Autodesk Inventor part; units mm, degrees
ref_plane "YZ Plane" through (0, 0, 0) normal (1, 0, 0) x (0, 1, 0)
ref_plane "XZ Plane" through (0, 0, 0) normal (0, 1, 0) x (-1, 0, 0)
ref_plane "XY Plane" through (0, 0, 0) normal (0, 0, 1) x (1, 0, 0)
sketch "Sketch1" plane through (0, 0, 0) normal (0, 0, 1) x (1, 0, 0)
  line L0 (0, 0) -> (25.4, 0)
  line L1 (25.4, 0) -> (25.4, 25.4)
  line L2 (25.4, 25.4) -> (0, 25.4)
  line L3 (0, 25.4) -> (0, 0)
  line L4 (3.175, 3.175) -> (22.225, 3.175)
  line L5 (22.225, 3.175) -> (22.225, 22.225)
  line L6 (22.225, 22.225) -> (3.175, 22.225)
  line L7 (3.175, 22.225) -> (3.175, 3.175)
  dimension "d0" = 25.4
  dimension "d1" = 25.4
  dimension "d2" = 19.05
  dimension "d3" = 19.05
  dimension "d4" = 3.175
  dimension "d5" = 3.175
extrude "Extrusion1" add sketch "Sketch1" along normal blind 146.05
sketch "Sketch2" plane through (0, 0, 0) normal (-1, 0, 0) x (0, 0, 1)
  line L0 (0, 25.4) -> (0, 0)
  line L1 (0, 0) -> (146.05, 0)
  point P0 (6.35, 12.7)
  point P1 (57.15, 12.7)
  dimension "d8" = 12.7
  dimension "d9" = 6.35
  dimension "d10" = 12.7
  dimension "d11" = 57.15
hole "Hole1" at (0, 12.7, 6.35) at (0, 12.7, 57.15) direction (1, 0, 0) diameter 6.35 end through all
sketch "Sketch3" plane through (25.4, 0, 0) normal (1, 0, 0) x (0, 0, -1)
  line L0 (-146.05, 0) -> (-146.05, 25.4)
  line L1 (0, 0) -> (-146.05, 0)
  point P0 (-95.25, 12.7)
  dimension "d19" = 50.8
  dimension "d20" = 12.7
hole "Hole2" at (25.4, 12.7, 95.25) direction (-1, 0, 0) diameter 17.4625 end through all
properties part number "back roller 1x1"
The model under review builds one solid part; all positions refer to its coordinate system, in mm. A direction names the side the tool comes from. Give positions to 0.01 mm unless a question says otherwise; leave off trailing zeros. Order: outer loops, then holes, each group sorted by start corner. A loop starts at its lowest first (then second) coordinate and runs counter-clockwise, first axis right, second up. Notation, with made-up numbers: M 71.5,75.5 L 111.5,75.5 A15 cw 111.5,79.5 Z; hole C 23.25,-32.5 d10. An arc over 180 degrees is marked long. Use one line per item in the form item = value. Start each with the question number.
Item 1: For faces 4 (the flat face through (13, 0, 72)), 5 (the flat face through (3.175, 13, 72)), list the 3-axis set-ups (+Z, -Z, +X, -X, +Y, -Y) from which the entire face can be reached by the end or side of a thin tool; tool diameter is ignored.
Item 2: We need section B-B on z = 95.25. Give the boundary of the cut face in (x, y) (3 decimals), plus the area to 3 significant figures.
Item 3: We need section A-A on x = 11. Give the boundary of the cut face in (y, z) (3 decimals), plus the area to 3 significant figures.
Item 4: Insertion check: pin 1 Ø8 at (x, z) = (18.5, 66) entering from -Y. The pin has a flat end and moves straight along its axis. Give the tip position at first contact, or say it passes through.
Item 5: We need section C-C on y = 12.7. Give the number of separate pieces and of enclosed holes in the cut face, plus the area to 3 significant figures.
Item 6: To check wall thickness, follow line 1 along Z through (x, y) = (0.8, 12.7) (3 decimals); line 2 along Y through (x, z) = (0.7, 6.35) (3 decimals); line 3 along X through (y, z) = (6, 127.5) (3 decimals). State the ranges of each line that lie inside material, in increasing order. Write a range as from..to.
Item 7: We need section D-D on z = 111.5. Give the boundary of the cut face in (x, y) (3 decimals).
Item 8: The part is to be moulded in two halves that separate along Z. For faces 1 (the flat face through (22.225, 13, 72)), 2 (the cylindrical face through (23.79, 16.044, 87.185)), 3 (the flat face through (24, 13, 146.05)), say which applies: pulls with the +Z half, pulls with the -Z half, needs draft (parallel to the pull), parting line crosses it, or undercut.
Completed:
q1.face_4 = +Z, -Z, +X, -X, -Y
q1.face_5 = +Z, -Z
q2.outline = M 0,0 L 25.4,0 L 25.4,3.969 L 22.225,3.969 L 22.225,3.175 L 3.175,3.175 L 3.175,3.969 L 0,3.969 Z; M 0,21.431 L 3.175,21.431 L 3.175,22.225 L 22.225,22.225 L 22.225,21.431 L 25.4,21.431 L 25.4,25.4 L 0,25.4 Z
q2.area = 171 mm²
q3.outline = M 0,0 L 3.175,0 L 3.175,146.05 L 0,146.05 Z; M 22.225,0 L 25.4,0 L 25.4,146.05 L 22.225,146.05 Z
q3.area = 927 mm²
q4.pin_1 = 0
q5.separate_pieces = 8
q5.enclosed_holes = 0
q5.area = 736 mm²
q6.line_1 = 0..3.175, 9.525..53.975, 60.325..86.519, 103.981..146.05
q6.line_2 = 0..9.525, 15.875..25.4
q6.line_3 = 0..3.175, 22.225..25.4
q7.outline = M 0,0 L 25.4,0 L 25.4,25.4 L 0,25.4 Z; hole M 3.175,3.175 L 22.225,3.175 L 22.225,22.225 L 3.175,22.225 Z
q8.face_1 = needs draft
q8.face_2 = undercut
q8.face_3 = pulls with the +Z half
